The listing builds one solid part. Answer for the finished solid, in the listing's coordinates (mm). Face numbers are marked on the shaded views. Coordinates: 2 decimals unless noted, no trailing zeros. Answer as a JSON object with one key per item and string values. Group by question number.
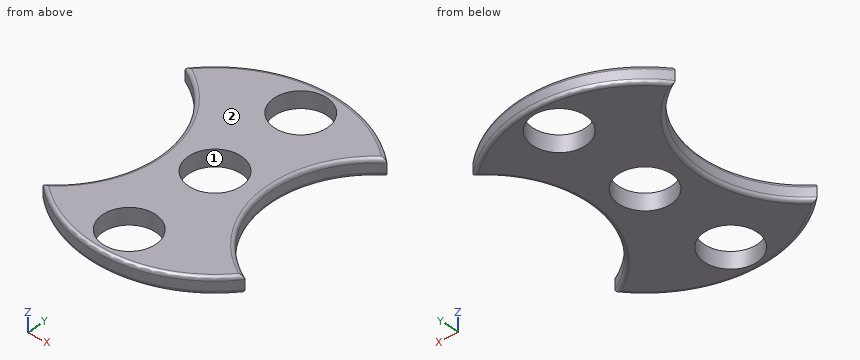
from build123d import *

# Parameters (mm, degrees)
F0_R     = 11.2
F1_DEPTH = 7
F2_R     = 1.5
F3_R     = 1.5


with BuildPart() as f1:
    # F0 (on Top) → F1 (new body)
    with BuildSketch(Plane.XY):
        with BuildLine():
            ThreePointArc((-42.542229, 33.110583), (-18.684815, -1.724094), (-35.765112, -40.336196))
            ThreePointArc((-35.765112, -40.336196), (4.953252, -53.680697), (42.542229, -33.110583))
            ThreePointArc((42.542229, -33.110583), (18.684815, 1.724094), (35.765112, 40.336196))
            ThreePointArc((35.765112, 40.336196), (-4.953252, 53.680697), (-42.542229, 33.110583))
        make_face()
        with Locations((0, -39.85231)):
            Circle(F0_R, mode=Mode.SUBTRACT)
        Circle(F0_R, mode=Mode.SUBTRACT)
        with Locations((0, 39.85231)):
            Circle(F0_R, mode=Mode.SUBTRACT)
    extrude(amount=F1_DEPTH)

    # F2
    f2_edges = [f1.edges().sort_by_distance(p)[0] for p in [
        (18.684815, 1.724094, 7),
        (4.953252, -53.680697, 7),
        (-18.684815, -1.724094, 7),
        (-4.953252, 53.680697, 7),
    ]]
    fillet(f2_edges, radius=F2_R)

    # F3
    f3_edges = [f1.edges().sort_by_distance(p)[0] for p in [
        (4.953252, -53.680697, 0),
        (18.684815, 1.724094, 0),
        (-4.953252, 53.680697, 0),
        (-18.684815, -1.724094, 0),
    ]]
    fillet(f3_edges, radius=F3_R)


solid = f1.part
Item 1: Consider L1, parallel to Y at x = 0, z = 5; L2, parallel to Y at x = 1.5, z = 6; L3, parallel to X at y = -9.5, z = 4.25. Determine where each line is inside the solid, lowest interval first. Write a range as from..to.
Item 2: Flat-ended cylindrical pins translate along their axes: pin 1 Ø4 at (x, z) = (24, 4.5) entering from -Y; pin 2 Ø3 at (y, z) = (4.5, 1.5) entering from -X; pin 3 Ø1 at (x, z) = (-23, 6) entering from -Y. Find the tip coordinate at first contact, or state that the pin passes through.
Item 3: For a pull along Y with two mould halves and no side action, classify the marked faces 1 and 2 as +Y half, -Y half, draft (parallel to the pull), parting line (faces both ways), or undercut.
Item 4: A cutting plane is placed at A-A, the plane x = 0. State how many separate pieces and enclosed holes the cut face has, and give its area (3 significant figures).
Answer:
{
 "1": {"L1": "-53.91..-51.05, -28.65..-11.2, 11.2..28.65, 51.05..53.91", "L2": "-53.8..-50.95, -28.75..-11.1, 11.1..28.75, 50.95..53.8", "L3": "-18.67..-5.93, 5.93..21.26"},
 "2": {"pin 1": "y = -49.22", "pin 2": "x = -20.11", "pin 3": "y = -48.94"},
 "3": {"face 1": "undercut", "face 2": "draft"},
 "4": {"separate pieces": "4", "enclosed holes": "0", "area": "282 mm2"}
}
